from build123d import *

# Parameters (mm, degrees)
BOSS_EXTRUDE1_DEPTH      = 25.4
BOSS_EXTRUDE1_DEPTH_BACK = 25.4
SKETCH1_R                = 50.8
CUT_EXTRUDE1_DEPTH       = 12.7
CUT_EXTRUDE2_START       = -12.7
CUT_EXTRUDE2_DEPTH       = 12.7
SKETCH5_R                = 12.7
BOSS_EXTRUDE2_DEPTH      = 6.35
BOSS_EXTRUDE3_START      = 6.35
SKETCH6_R                = 12.7
BOSS_EXTRUDE3_DEPTH      = 6.35
SKETCH7_R                = 6.35
CUT_EXTRUDE3_DEPTH       = 96.882897328
FILLET1_R                = 5
FILLET2_R                = 1


with BuildPart() as part:
    # Sketch1 → Boss-Extrude1 (new, two sides: drawn at the far end of the back side and taken through both)
    with BuildSketch(Plane.XY.offset(-BOSS_EXTRUDE1_DEPTH_BACK)):
        Circle(SKETCH1_R)
    extrude(amount=BOSS_EXTRUDE1_DEPTH + BOSS_EXTRUDE1_DEPTH_BACK)

    # Sketch3 → Cut-Extrude1 (cut)
    with BuildSketch(Plane.XY.offset(25.4)):
        with BuildLine():
            Line((-19.247414599, -36.5125), (-8.117054136, -17.234150172))
            ThreePointArc((-8.117054136, -17.234150172), (0, -19.05), (8.117054136, -17.234150172))
            Line((8.117054136, -17.234150172), (19.247414599, -36.5125))
            ThreePointArc((19.247414599, -36.5125), (0, -41.275), (-19.247414599, -36.5125))
        make_face()
        with BuildLine():
            Line((-21.997045256, -34.925), (-10.866684793, -15.646650172))
            ThreePointArc((-10.866684793, -15.646650172), (-16.497783942, -9.525), (-18.98373893, -1.5875))
            Line((-18.98373893, -1.5875), (-41.244459855, -1.5875))
            ThreePointArc((-41.244459855, -1.5875), (-35.745198541, -20.6375), (-21.997045256, -34.925))
        make_face()
        with BuildLine():
            Line((21.997045256, -34.925), (10.866684793, -15.646650172))
            ThreePointArc((10.866684793, -15.646650172), (16.497783942, -9.525), (18.98373893, -1.5875))
            Line((18.98373893, -1.5875), (41.244459855, -1.5875))
            ThreePointArc((41.244459855, -1.5875), (35.745198541, -20.6375), (21.997045256, -34.925))
        make_face()
        with BuildLine():
            Line((-21.997045256, 34.925), (-10.866684793, 15.646650172))
            ThreePointArc((-10.866684793, 15.646650172), (-16.497783942, 9.525), (-18.98373893, 1.5875))
            Line((-18.98373893, 1.5875), (-41.244459855, 1.5875))
            ThreePointArc((-41.244459855, 1.5875), (-35.745198541, 20.6375), (-21.997045256, 34.925))
        make_face()
        with BuildLine():
            Line((41.244459855, 1.5875), (18.98373893, 1.5875))
            ThreePointArc((18.98373893, 1.5875), (16.497783942, 9.525), (10.866684793, 15.646650172))
            Line((10.866684793, 15.646650172), (21.997045256, 34.925))
            ThreePointArc((21.997045256, 34.925), (35.745198541, 20.6375), (41.244459855, 1.5875))
        make_face()
        with BuildLine():
            Line((-8.117054136, 17.234150172), (-19.247414599, 36.5125))
            ThreePointArc((-19.247414599, 36.5125), (0, 41.275), (19.247414599, 36.5125))
            Line((19.247414599, 36.5125), (8.117054136, 17.234150172))
            ThreePointArc((8.117054136, 17.234150172), (0, 19.05), (-8.117054136, 17.234150172))
        make_face()
    extrude(amount=-CUT_EXTRUDE1_DEPTH, mode=Mode.SUBTRACT)

    # Sketch4 → Cut-Extrude2 (cut)
    with BuildSketch(Plane(origin=(0, 0, -25.4), x_dir=(-1, 0, 0), z_dir=(0, 0, -1)).offset(CUT_EXTRUDE2_START)):
        with BuildLine():
            Line((21.997045256, -34.925), (10.866684793, -15.646650172))
            ThreePointArc((10.866684793, -15.646650172), (16.497783942, -9.525), (18.98373893, -1.5875))
            Line((18.98373893, -1.5875), (41.244459855, -1.5875))
            ThreePointArc((41.244459855, -1.5875), (35.745198541, -20.6375), (21.997045256, -34.925))
        make_face()
        with BuildLine():
            Line((8.117054136, -17.234150172), (19.247414599, -36.5125))
            ThreePointArc((19.247414599, -36.5125), (0, -41.275), (-19.247414599, -36.5125))
            Line((-19.247414599, -36.5125), (-8.117054136, -17.234150172))
            ThreePointArc((-8.117054136, -17.234150172), (0, -19.05), (8.117054136, -17.234150172))
        make_face()
        with BuildLine():
            Line((-10.866684793, -15.646650172), (-21.997045256, -34.925))
            ThreePointArc((-21.997045256, -34.925), (-35.745198541, -20.6375), (-41.244459855, -1.5875))
            Line((-41.244459855, -1.5875), (-18.98373893, -1.5875))
            ThreePointArc((-18.98373893, -1.5875), (-16.497783942, -9.525), (-10.866684793, -15.646650172))
        make_face()
        with BuildLine():
            Line((-21.997045256, 34.925), (-10.866684793, 15.646650172))
            ThreePointArc((-10.866684793, 15.646650172), (-16.497783942, 9.525), (-18.98373893, 1.5875))
            Line((-18.98373893, 1.5875), (-41.244459855, 1.5875))
            ThreePointArc((-41.244459855, 1.5875), (-35.745198541, 20.6375), (-21.997045256, 34.925))
        make_face()
        with BuildLine():
            Line((41.244459855, 1.5875), (18.98373893, 1.5875))
            ThreePointArc((18.98373893, 1.5875), (16.497783942, 9.525), (10.866684793, 15.646650172))
            Line((10.866684793, 15.646650172), (21.997045256, 34.925))
            ThreePointArc((21.997045256, 34.925), (35.745198541, 20.6375), (41.244459855, 1.5875))
        make_face()
        with BuildLine():
            Line((-8.117054136, 17.234150172), (-19.247414599, 36.5125))
            ThreePointArc((-19.247414599, 36.5125), (0, 41.275), (19.247414599, 36.5125))
            Line((19.247414599, 36.5125), (8.117054136, 17.234150172))
            ThreePointArc((8.117054136, 17.234150172), (0, 19.05), (-8.117054136, 17.234150172))
        make_face()
    extrude(amount=CUT_EXTRUDE2_DEPTH, mode=Mode.SUBTRACT)

    # Sketch5 → Boss-Extrude2 (add)
    with BuildSketch(Plane(origin=(0, 0, -25.4), x_dir=(-1, 0, 0), z_dir=(0, 0, -1))):
        with Locations(Location((0, 0, 0), (0, 0, 180))):
            Circle(SKETCH5_R)
    extrude(amount=BOSS_EXTRUDE2_DEPTH)

    # Sketch6 → Boss-Extrude3 (add)
    with BuildSketch(Plane.XY.offset(25.4).offset(BOSS_EXTRUDE3_START)):
        Circle(SKETCH6_R)
    extrude(amount=-BOSS_EXTRUDE3_DEPTH)

    # Sketch7 → Cut-Extrude3 (cut, through all)
    with BuildSketch(Plane.XY.offset(31.75)):
        Circle(SKETCH7_R)
    extrude(amount=-CUT_EXTRUDE3_DEPTH, mode=Mode.SUBTRACT)

    # Fillet1
    fillet1_edges = [part.edges().sort_by_distance(p)[0] for p in [
        (-50.8, 0, -25.4),
        (-50.8, 0, 25.4),
    ]]
    fillet(fillet1_edges, radius=FILLET1_R)

    # Fillet2
    fillet2_edges = [part.edges().sort_by_distance(p)[0] for p in [
        (0, -19.05, -25.4),
        (16.497783942, 9.525, -25.4),
        (-16.497783942, 9.525, -25.4),
        (0, 19.05, -25.4),
        (-16.497783942, -9.525, -25.4),
        (0, -19.05, 25.4),
        (16.497783942, 9.525, 25.4),
        (16.497783942, -9.525, 25.4),
        (0, 19.05, 25.4),
        (-16.497783942, -9.525, 25.4),
        (-16.497783942, 9.525, 25.4),
        (16.497783942, -9.525, -25.4),
    ]]
    fillet(fillet2_edges, radius=FILLET2_R)


solid = part.part
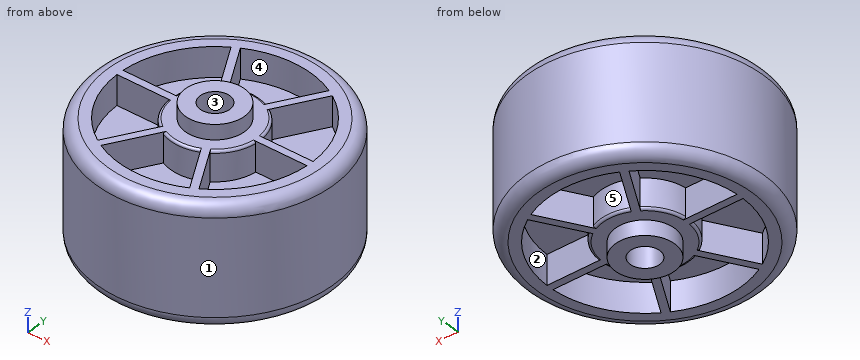
Part model, mm, in its own coordinate system. Face numbers are marked on the shaded views. A direction names the side the tool comes from. Coordinates: 2 decimals unless noted, no trailing zeros. Loops run counter-clockwise (first coordinate to the right, second up) from the corner with the lowest first, then second, coordinate; pieces in that order, holes last. Notation, with made-up numbers: M -19,54.5 L 14,54.5 A23 ccw 14,68.5 Z; hole C 53.5,69.25 d5. An arc over 180 degrees is marked long. Use a Markdown table: item, result. Add a question column.
Q1. Which spindle directions (+Z, -Z, +X, -X, +Y, -Y) get a long thin tool onto all of the face, cutting with end or side? Do the marked faces 3, 4 and 5. Say none if no direction does.
Q2. Cut at B-B (z = 17). Give the number of separate pieces and of enclosed holes in the cut face, and give its area (3 significant figures).
Q3. Cut at A-A (y = 0). Write the cut outline in (x, z), and give its area (3 significant figures).
Q4. Probe L1, parallel to Y at x = -9.5, z = -15; L2, parallel to Y at x = 36, z = -23; L3, parallel to Y at x = 0, z = -5. List the from-to ranges inside material, lowest first.
Q5. Cut at C-C (z = -9.5). Write the cut outline in (x, y), and give its area (3 significant figures).
Q6. Pin check, flat tips, straight feed: P1, Ø14, axis at x = 35, z = -18, coming from the -Y side; P2, Ø12, axis at x = -0.5, y = -28.5, coming from the -Z side; P3, Ø4, axis at y = -21, z = -20.5, coming from the +X side. Stop position of each tip, or through.
Q7. Mould opens along X. For the marked faces 1 and 2 say: +X half, -X half, draft (parallel to the pull), parting line (faces both ways), or undercut.
Worked out:
| question | item | result |
|---|---|---|
| 1 | face 3 | +Z, -Z |
| 1 | face 4 | +Z |
| 1 | face 5 | -Z |
| 2 | separate pieces | 1 |
| 2 | enclosed holes | 7 |
| 2 | area | 4,190 mm2 |
| 3 | outline | M -50.8,-20.4 A5 ccw -45.8,-25.4 L -12.7,-25.4 L -12.7,-31.75 L -6.35,-31.75 L -6.35,31.75 L -12.7,31.75 L -12.7,25.4 L -45.8,25.4 A5 ccw -50.8,20.4 Z; M 6.35,-31.75 L 12.7,-31.75 L 12.7,-25.4 L 45.8,-25.4 A5 ccw 50.8,-20.4 L 50.8,20.4 A5 ccw 45.8,25.4 L 12.7,25.4 L 12.7,31.75 L 6.35,31.75 Z |
| 3 | area | 4,660 mm2 |
| 4 | L1 | y = -49.9 to -40.17, -19.63 to 19.63, 40.17 to 49.9 |
| 4 | L2 | y = -34.8 to -20.19, -1.59 to 1.59, 20.19 to 34.8 |
| 4 | L3 | y = -50.8 to -6.35, 6.35 to 50.8 |
| 5 | outline | C 0,0 d101.6; hole C 0,0 d12.7 |
| 5 | area | 7,980 mm2 |
| 6 | P1 | stops at y = -42.39 |
| 6 | P2 | stops at z = -12.7 |
| 6 | P3 | stops at x = 47.11 |
| 7 | face 1 | parting line |
| 7 | face 2 | undercut |
